Can you work these out from the model? Positions are in its coordinate system, mm. A direction names the side the tool comes from. Give positions to 0.01 mm unless a question says otherwise; leave off trailing zeros. Loops run counter-clockwise (first coordinate to the right, second up) from the corner with the lowest first, then second, coordinate; pieces in that order, holes last.
from build123d import *

# Parameters (mm, degrees)
SKETCH_1_W      = 32
SKETCH_1_H      = 32
SKETCH_1_R      = 1
EXTRUDE_1_DEPTH = 1.6
SKETCH_2_W      = 16
SKETCH_2_H      = 16
EXTRUDE_2_DEPTH = 6.5
SKETCH_3_R      = 6.75
EXTRUDE_3_DEPTH = 9


with BuildPart() as part:
    # 草图1 → 凸台-拉伸1 (new body)
    with BuildSketch(Plane(origin=(0, 0, 0), x_dir=(1, 0, 0), z_dir=(0, 1, 0))):
        Rectangle(SKETCH_1_W, SKETCH_1_H)
        with Locations(Location((13.5, 13.5, 0), (0, 0, 270))):
            Circle(SKETCH_1_R, mode=Mode.SUBTRACT)
        with Locations(Location((-13.5, -13.5, 0), (0, 0, 90))):
            Circle(SKETCH_1_R, mode=Mode.SUBTRACT)
        with Locations(Location((-13.5, 13.5, 0), (0, 0, 270))):
            Circle(SKETCH_1_R, mode=Mode.SUBTRACT)
        with Locations(Location((13.5, -13.5, 0), (0, 0, 90))):
            Circle(SKETCH_1_R, mode=Mode.SUBTRACT)
    extrude(amount=EXTRUDE_1_DEPTH)

    # 草图2 → 凸台-拉伸2 (add)
    with BuildSketch(Plane.XZ):
        Rectangle(SKETCH_2_W, SKETCH_2_H)
        with BuildLine():
            Line((-10, -2), (-8, -2))
            Line((-8, -2), (-8, 2))
            Line((-8, 2), (-10, 2))
            ThreePointArc((-10, 2), (-12, 0), (-10, -2))
        make_face()
        with BuildLine():
            Line((8, 2), (8, -2))
            Line((8, -2), (10, -2))
            ThreePointArc((10, -2), (12, 0), (10, 2))
            Line((10, 2), (8, 2))
        make_face()
    extrude(amount=EXTRUDE_2_DEPTH)

    # 草图3 → 凸台-拉伸3 (add)
    with BuildSketch(Plane.XZ.offset(6.5)):
        with Locations(Location((0, 0, 0), (0, 0, 270))):
            Circle(SKETCH_3_R)
    extrude(amount=EXTRUDE_3_DEPTH)


solid = part.part
(1) Suppose I cut it at C-C on x = -13.5. List the corners of the cut face in (y, z) for me.
Returned:
outline: (0, -16) - (1.6, -16) - (1.6, -14.5) - (0, -14.5) - close; (0, -12.5) - (1.6, -12.5) - (1.6, 12.5) - (0, 12.5) - close; (0, 14.5) - (1.6, 14.5) - (1.6, 16) - (0, 16) - close
(2) Which directions (+Z, -Z, +X, -X, +Y, -Y) give clear straight access to the entire face, cutting with the end or side of a thin tool? Please do faces 1 (the flat face through (-9, -3, 2)), 2 (the flat face through (-8, -3, -5)), 3 (the flat face through (9, -3, -2)), 4 (the flat face through (9, -3, 2)).
Returned:
face 1: +Z, -X, -Y
face 2: -Z, -X, -Y
face 3: -Z, +X, -Y
face 4: +Z, +X, -Y
(3) Will these pins go through, and if not, where does the flat tip stop? P1, Ø2, axis at x = -9.5, y = -2, coming from the -Z side; P2, Ø1.8, axis at y = -4.5, z = -3.5, coming from the -X side; P3, Ø5, axis at y = -8, z = 2, coming from the +X side.
Returned:
P1: stops at z = -2
P2: stops at x = -8
P3: stops at x = 12
(4) Thinking about a two-plate mould opening in Z: for faces 5 (the flat face through (0, 0, -11)), 6 (the flat face through (0, -3, 8)), 7 (the cylindrical face through (-12.61, 0.79, 13.04)), 8 (the flat face through (0, 1, -16)), which applies, pulls with the +Z half, pulls with the -Z half, needs draft (parallel to the pull), parting line crosses it, or undercut?
Returned:
face 5: needs draft
face 6: pulls with the +Z half
face 7: undercut
face 8: pulls with the -Z half
(5) Suppose I cut it at B-B on z = -14. List the corners of the cut face in (x, y) for me.
Returned:
outline: (-16, 0) - (-14.37, 0) - (-14.37, 1.6) - (-16, 1.6) - close; (-12.63, 0) - (12.63, 0) - (12.63, 1.6) - (-12.63, 1.6) - close; (14.37, 0) - (16, 0) - (16, 1.6) - (14.37, 1.6) - close
(6) Suppose I cut it at A-A on y = -3.25. List the corners of the cut face in (x, z) for me, plus the area to 3 significant figures.
Returned:
outline: (-10, -2) - (-8, -2) - (-8, -8) - (8, -8) - (8, -2) - (10, -2) arc R2 ccw to (10, 2) - (8, 2) - (8, 8) - (-8, 8) - (-8, 2) - (-10, 2) arc R2 ccw to start
area: 285 mm2
(7) Suppose I cut it at D-D on z = 0. List the corners of the cut face in (x, y) for me.
Returned:
outline: (-16, 0) - (-12, 0) - (-12, -6.5) - (-6.75, -6.5) - (-6.75, -15.5) - (6.75, -15.5) - (6.75, -6.5) - (12, -6.5) - (12, 0) - (16, 0) - (16, 1.6) - (-16, 1.6) - close
(8) Please list where these lines run through material, in increasing order: probe 1 along X at (y, z) = (0.6, 13.5); probe 2 along Y at (x, z) = (-11, -5.5); probe 3 along Z at (x, y) = (-8.5, -3.5).
Returned:
probe 1: x = -16 to -14.5, -12.5 to 12.5, 14.5 to 16
probe 2: y = 0 to 1.6
probe 3: z = -2 to 2
